CAD build for the part. Positions are in the model's coordinates, mm. Face numbers are marked on the shaded views. A direction names the side the tool comes from. Give positions to 0.01 mm unless a question says otherwise; leave off trailing zeros. Order: outer loops, then holes, each group sorted by start corner. A loop starts at its lowest first (then second) coordinate and runs counter-clockwise, first axis right, second up.
Item 1: Flat gauge pins, fed straight in: P1, Ø4, axis at y = 0.5, z = -1, coming from the -X side; P2, Ø1.5, axis at x = 17.5, z = -10, coming from the +Y side; P3, Ø3, axis at x = -20.35, y = -8.15, coming from the -Z side; P4, Ø6, axis at x = 9, y = 6, coming from the -Z side. Where does each tip first touch, or does it go through?
Item 2: Band-saw the part on D-D on z = -10. Give the cut face in (x, y).
Item 3: Band-saw the part on C-C on z = 1.5. Give the cut face in (x, y).
Item 4: Which spindle directions (+Z, -Z, +X, -X, +Y, -Y) get a long thin tool onto all of the face, cutting with end or side? Do the marked faces 4, 5 and 6. Say none if no direction does.
Item 5: Two-plate mould, pull along Y, no slides. Class the marked faces 1, 2 and 3: released by +Y, released by -Y, zero draft, split by the parting line, or undercut.
Item 6: Band-saw the part on A-A on x = 13.45. Give the cut face in (y, z), plus the area to 3 significant figures.
Item 7: Band-saw the part on B-B on y = 0. Give the cut face in (x, z), plus the area to 3 significant figures.
Item 8: Wall check: L1, parallel to Y at x = -11.85, z = 1.3; L2, parallel to X at y = -11.5, z = -10; L3, parallel to X at y = -1.5, z = 0.5. Give the ranges that are in metal, low to high.
```python
from build123d import *

# Parameters (mm, degrees)
SKETCH_1_W          = 45.7
SKETCH_1_H          = 21.3
EXTRUDE_1_DEPTH     = 5
SKETCH_2_R          = 1.55
SKETCH_2_R_2        = 8.5
CUT_EXTRUDE_1_DEPTH = 13.95
SKETCH_7_W          = 45.7
SKETCH_7_H          = 20
EXTRUDE_3_DEPTH     = 3
SKETCH_3_W          = 10.7
SKETCH_3_H          = 2.5
CUT_EXTRUDE_2_DEPTH = 13.95
FILLET_4_R          = 0.5
SKETCH_11_R         = 2
CUT_EXTRUDE_4_DEPTH = 3
FILLET_5_R          = 0.5


with BuildPart() as part:
    # 草圖1 → 填料-伸長1 (new body)
    with BuildSketch(Plane.XY):
        Rectangle(SKETCH_1_W, SKETCH_1_H)
    extrude(amount=EXTRUDE_1_DEPTH)

    # 草圖2 → 除料-伸長1 (cut)
    with BuildSketch(Plane.XY.offset(5)):
        with Locations((-20.35, -8.15)):
            Circle(SKETCH_2_R)
        with Locations((20.35, 8.15)):
            Circle(SKETCH_2_R)
        with Locations((-11.85, 0)):
            Circle(SKETCH_2_R_2)
        with Locations((13.45, 0)):
            Circle(SKETCH_2_R_2)
    extrude(amount=-CUT_EXTRUDE_1_DEPTH, mode=Mode.SUBTRACT)

    # 草圖7 → 填料-伸長3 (add)
    with BuildSketch(Plane.XZ.offset(10.65)):
        with Locations((0, -5)):
            Rectangle(SKETCH_7_W, SKETCH_7_H)
    extrude(amount=EXTRUDE_3_DEPTH)

    # 草圖3 → 除料-伸長2 (cut)
    with BuildSketch(Plane.XY.offset(5)):
        with Locations((0.5, 9.4)):
            Rectangle(SKETCH_3_W, SKETCH_3_H)
    extrude(amount=-CUT_EXTRUDE_2_DEPTH, mode=Mode.SUBTRACT)

    # 圓角4
    fillet_4_edges = [part.edges().sort_by_distance(p)[0] for p in [
        (14.35, 10.65, 5),
        (5.85, 10.65, 2.5),
        (14.35, 10.65, 0),
        (-13.85, 10.65, 0),
        (-4.85, 10.65, 2.5),
        (-13.85, 10.65, 5),
        (-22.85, 10.65, 2.5),
        (-22.85, -1.5, 5),
        (-22.85, -13.65, -5),
        (-22.85, -12.15, -15),
        (-22.85, -10.65, -7.5),
        (-22.85, 0, 0),
        (22.85, -10.65, -7.5),
        (22.85, -12.15, -15),
        (22.85, -13.65, -5),
        (22.85, -1.5, 5),
        (22.85, 10.65, 2.5),
        (22.85, 0, 0),
    ]]
    fillet(fillet_4_edges, radius=FILLET_4_R)

    # 草圖11 → 除料-伸長4 (cut)
    with BuildSketch(Plane(origin=(0, -10.65, 0), x_dir=(1, 0, 0), z_dir=(0, 1, 0))):
        with Locations(Location((0, 10, 0), (0, 0, 270))):
            Circle(SKETCH_11_R)
        with Locations(Location((16, 10, 0), (0, 0, 270))):
            Circle(SKETCH_11_R)
        with Locations(Location((-16, 10, 0), (0, 0, 270))):
            Circle(SKETCH_11_R)
    extrude(amount=-CUT_EXTRUDE_4_DEPTH, mode=Mode.SUBTRACT)

    # 圓角5
    # the kernel refuses this fillet: 0.5 mm, written as the material it takes off along each edge
    with BuildSketch(Plane(origin=(-22.35, -13.15, -14.5), x_dir=(0, 0, -1), z_dir=(0, -1, 0))) as fillet_5_piece_1_section:
        Polygon((0, 0), (FILLET_5_R, 0), (FILLET_5_R, -FILLET_5_R), (0, -FILLET_5_R), align=None)
    fillet_5_piece_1 = extrude(amount=FILLET_5_R, mode=Mode.PRIVATE)
    fillet_5_piece_1 = fillet_5_piece_1 - Plane(origin=(-22.35, -13.15, -14.5), x_dir=(0.7071067811865475, 0, 0.7071067811865475), z_dir=(0, -1, 0)) * Sphere(FILLET_5_R, mode=Mode.PRIVATE)
    add(fillet_5_piece_1, mode=Mode.SUBTRACT)
    with BuildSketch(Plane(origin=(-22.35, -11.15, -14.5), x_dir=(0, 0, -1), z_dir=(0, 1, 0))) as fillet_5_piece_2_section:
        Polygon((0, 0), (FILLET_5_R, 0), (FILLET_5_R, FILLET_5_R), (0, FILLET_5_R), align=None)
    fillet_5_piece_2 = extrude(amount=FILLET_5_R, mode=Mode.PRIVATE)
    fillet_5_piece_2 = fillet_5_piece_2 - Plane(origin=(-22.35, -11.15, -14.5), x_dir=(0.7071067811865475, 0, 0.7071067811865475), z_dir=(0, 1, 0)) * Sphere(FILLET_5_R, mode=Mode.PRIVATE)
    add(fillet_5_piece_2, mode=Mode.SUBTRACT)
    with BuildSketch(Plane(origin=(22.35, -11.15, -14.5), x_dir=(0, 0, -1), z_dir=(0, 1, 0))) as fillet_5_piece_3_section:
        Polygon((0, 0), (FILLET_5_R, 0), (FILLET_5_R, -FILLET_5_R), (0, -FILLET_5_R), align=None)
    fillet_5_piece_3 = extrude(amount=FILLET_5_R, mode=Mode.PRIVATE)
    fillet_5_piece_3 = fillet_5_piece_3 - Plane(origin=(22.35, -11.15, -14.5), x_dir=(-0.7071067811865475, 0, 0.7071067811865475), z_dir=(0, 1, 0)) * Sphere(FILLET_5_R, mode=Mode.PRIVATE)
    add(fillet_5_piece_3, mode=Mode.SUBTRACT)
    with BuildSketch(Plane(origin=(22.35, -13.15, -14.5), x_dir=(0, 0, -1), z_dir=(0, -1, 0))) as fillet_5_piece_4_section:
        Polygon((0, 0), (FILLET_5_R, 0), (FILLET_5_R, FILLET_5_R), (0, FILLET_5_R), align=None)
    fillet_5_piece_4 = extrude(amount=FILLET_5_R, mode=Mode.PRIVATE)
    fillet_5_piece_4 = fillet_5_piece_4 - Plane(origin=(22.35, -13.15, -14.5), x_dir=(-0.7071067811865475, 0, 0.7071067811865475), z_dir=(0, -1, 0)) * Sphere(FILLET_5_R, mode=Mode.PRIVATE)
    add(fillet_5_piece_4, mode=Mode.SUBTRACT)
    with BuildSketch(Plane(origin=(-22.35, -13.65, -15), x_dir=(0, 0, 1), z_dir=(1, 0, 0))) as fillet_5_piece_5:
        with BuildLine():
            CenterArc((FILLET_5_R, -FILLET_5_R), FILLET_5_R, 90, 90)
            Line((0, -FILLET_5_R), (0, 0))
            Line((0, 0), (FILLET_5_R, 0))
        make_face()
    extrude(amount=44.7, mode=Mode.SUBTRACT)
    with BuildSketch(Plane(origin=(-22.35, -10.65, -15), x_dir=(0, 0, 1), z_dir=(1, 0, 0))) as fillet_5_piece_6:
        with BuildLine():
            CenterArc((FILLET_5_R, FILLET_5_R), FILLET_5_R, 180, 90)
            Line((0, FILLET_5_R), (0, 0))
            Line((0, 0), (FILLET_5_R, 0))
        make_face()
    extrude(amount=44.7, mode=Mode.SUBTRACT)


solid = part.part
```
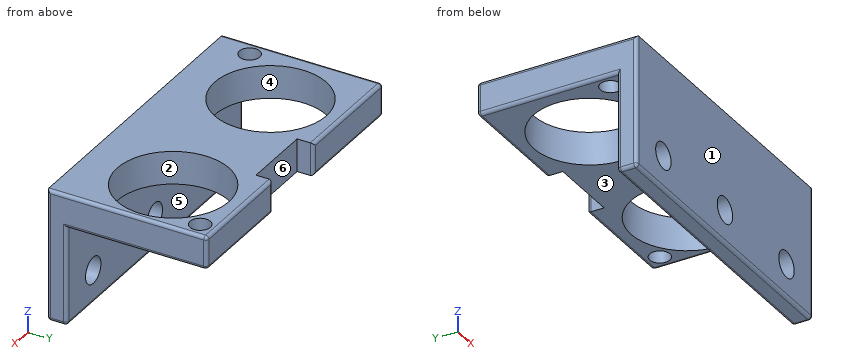
The answers:
1. P1: stops at x = -22.85
1. P2: stops at y = -10.65
1. P3: passes through
1. P4: stops at z = 0
2. outline: (-22.85, -13.15) arc R0.5 ccw to (-22.35, -13.65) - (-18, -13.65) - (-18, -10.65) - (-22.35, -10.65) arc R0.5 ccw to (-22.85, -11.15) - close; (-14, -13.65) - (-2, -13.65) - (-2, -10.65) - (-14, -10.65) - close; (2, -13.65) - (14, -13.65) - (14, -10.65) - (2, -10.65) - close; (18, -13.65) - (22.35, -13.65) arc R0.5 ccw to (22.85, -13.15) - (22.85, -11.15) arc R0.5 ccw to (22.35, -10.65) - (18, -10.65) - close
3. outline: (-22.85, -13.15) arc R0.5 ccw to (-22.35, -13.65) - (22.35, -13.65) arc R0.5 ccw to (22.85, -13.15) - (22.85, 10.15) arc R0.5 ccw to (22.35, 10.65) - (6.35, 10.65) arc R0.5 ccw to (5.85, 10.15) - (5.85, 8.15) - (-4.85, 8.15) - (-4.85, 10.15) arc R0.5 ccw to (-5.35, 10.65) - (-22.35, 10.65) arc R0.5 ccw to (-22.85, 10.15) - close; hole circle Ø3.1 at (-20.35, -8.15); hole circle Ø17 at (-11.85, 0); hole circle Ø17 at (13.45, 0); hole circle Ø3.1 at (20.35, 8.15)
4. face 4: +Z, -Z
4. face 5: -Z, +X, -X, +Y
4. face 6: +Z, -Z, +Y
5. face 1: released by -Y
5. face 2: undercut
5. face 3: zero draft
6. outline: (-13.65, -14.5) arc R0.5 ccw to (-13.15, -15) - (-11.15, -15) arc R0.5 ccw to (-10.65, -14.5) - (-10.65, 0) - (-8.5, 0) - (-8.5, 5) - (-13.65, 5) - close; (8.5, 0) - (10.15, 0) arc R0.5 ccw to (10.65, 0.5) - (10.65, 4.5) arc R0.5 ccw to (10.15, 5) - (8.5, 5) - close
6. area: 81.3 mm2
7. outline: (-22.85, 0.5) arc R0.5 ccw to (-22.35, 0) - (-20.35, 0) - (-20.35, 5) - (-22.35, 5) arc R0.5 ccw to (-22.85, 4.5) - close; (-3.35, 0) - (4.95, 0) - (4.95, 5) - (-3.35, 5) - close; (21.95, 0) - (22.35, 0) arc R0.5 ccw to (22.85, 0.5) - (22.85, 4.5) arc R0.5 ccw to (22.35, 5) - (21.95, 5) - close
7. area: 58.3 mm2
8. L1: y = -13.65 to -8.5, 8.5 to 10.65
8. L2: x = -22.85 to -18, -14 to -2, 2 to 14, 18 to 22.85
8. L3: x = -22.85 to -20.22, -3.48 to 5.08, 21.82 to 22.85
